For this review, use the dimensioned drawing (mm, ordinates from the lowest corner) and the shaded views. A direction names the side the tool comes from. Coordinates: 2 decimals unless noted, no trailing zeros. Loops run counter-clockwise (first coordinate to the right, second up) from the corner with the lowest first, then second, coordinate; pieces in that order, holes last. Notation, with made-up numbers: M -36.5,-16 L 1.5,-16 A19 ccw 1.5,-12 Z; hole C 20,-4 d2. An arc over 180 degrees is marked long. One line per item, written item: value.
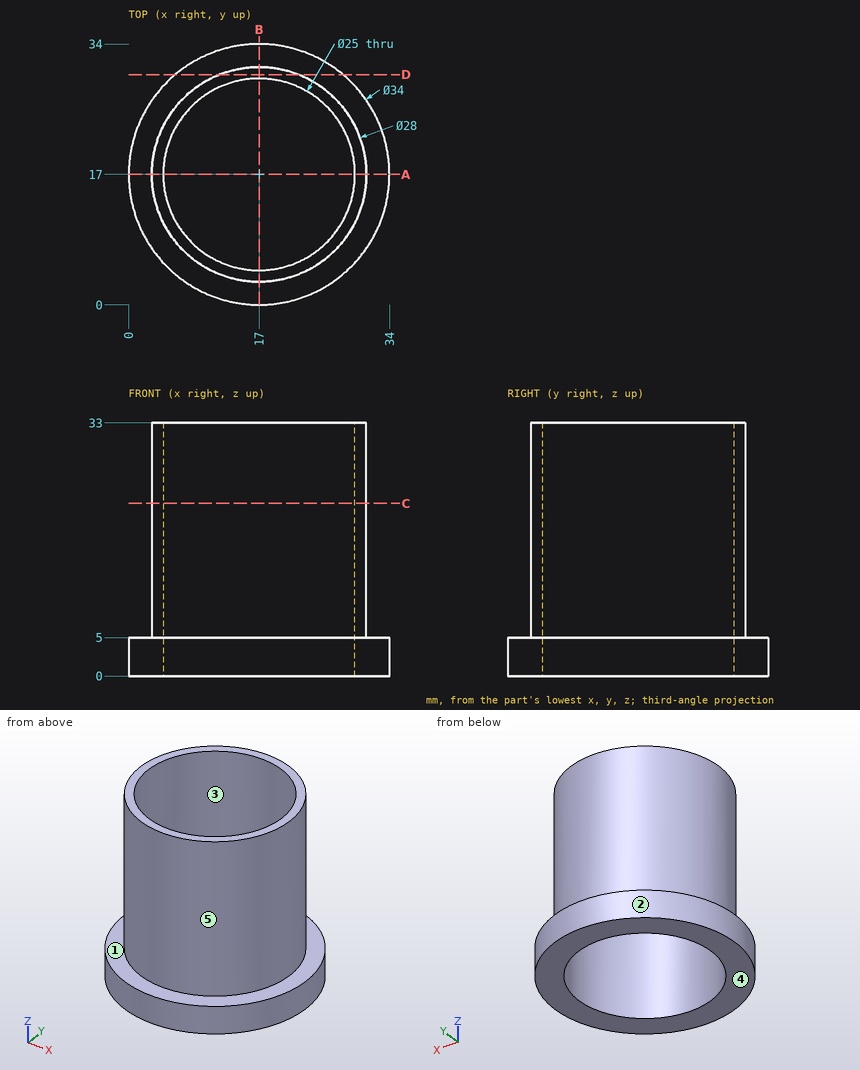
(1) Mouldability with a two-part tool opening along X and no side actions: class the marked faces 3, 4 and 5 as released by +X, released by -X, zero draft, split by the parting line, or undercut.
Reply:
face 3: undercut
face 4: zero draft
face 5: split by the parting line
(2) We need section D-D on y = 30. State the section outline as (x, z) points.
Reply:
outline: M 6.05,0 L 27.95,0 L 27.95,5 L 22.2,5 L 22.2,33 L 11.8,33 L 11.8,5 L 6.05,5 Z
(3) Tool access review of the marked faces 1 and 2: name each direction out of +Z, -Z, +X, -X, +Y, -Y from which nothing blocks a thin tool from reaching the whole face with its end or side.
Reply:
face 1: +Z
face 2: +Z, -Z
(4) We need section A-A on y = 17. State the section outline as (x, z) points.
Reply:
outline: M 0,0 L 4.5,0 L 4.5,33 L 3,33 L 3,5 L 0,5 Z; M 29.5,0 L 34,0 L 34,5 L 31,5 L 31,33 L 29.5,33 Z
(5) To check wall thickness, follow line 1 along Y through (x, z) = (17, 24); line 2 along Z through (x, y) = (30, 10); line 3 along Y through (x, z) = (23, 16). State the ranges of each line that lie inside material, in increasing order. Write a range as [from, to].
Reply:
line 1: y = [3, 4.5], [29.5, 31]
line 2: z = [0, 5]
line 3: y = [4.35, 6.03], [27.97, 29.65]
(6) Insertion check: pin 1 (4 mm diameter, centred on x = 6, z = 29.5, fed in from -Y); pin 2 (1 mm diameter, centred on y = 6, z = 7.5, fed in from +X); pin 3 (3 mm diameter, centred on x = 9, z = 6, fed in from -Y). Each pin has a flat end and moves straight along its axis. Give the tip position at first contact, or say it passes through.
Reply:
pin 1: stops at y = 6.28
pin 2: stops at x = 26.26
pin 3: stops at y = 1.46
(7) We need section C-C on z = 22.5. State the section outline as (x, y) points.
Reply:
outline: C 17,17 d28; hole C 17,17 d25
